Build history of the part. All positions in model axes, mm. A direction names the side the tool comes from. Give positions to 0.01 mm unless a question says otherwise; leave off trailing zeros. Loops run counter-clockwise (first coordinate to the right, second up) from the corner with the lowest first, then second, coordinate; pieces in that order, holes last.
1) Band-saw the part on C-C on x = 26. List the corners of the cut face in (y, z), then the cut area to 3 significant figures.
2) 3-axis set-ups, long thin cutter, end or side, ignore diameter. For faces 1 (the flat face through (5, 27, 5)), 2 (the cylindrical face through (-34.464, -14.013, 1.014)), 3 (the flat face through (-4, -27, 8)): which of +Z, -Z, +X, -X, +Y, -Y reach the whole face in a straight line?
3) Band-saw the part on A-A on y = 0. List the corners of the cut face in (x, z), then the cut area to 3 significant figures.
4) Flat gauge pins, fed straight in: P1, Ø0.7, axis at y = -27.5, z = 4.5, coming from the +X side; P2, Ø3, axis at x = 15.33, y = 32.57, coming from the +Z side; P3, Ø10, axis at x = -13, y = -23.5, coming from the +Z side. Where does each tip first touch, or does it go through?
5) Two-plate mould, pull along X, no slides. Class faces 4 (the flat face through (-2, 22, 9)), 5 (the cylindrical face through (-30.392, 16.864, 1.014)): +X half, -X half, draft (parallel to the pull), parting line (faces both ways), or undercut.
6) Band-saw the part on B-B on x = -7. List the corners of the cut face in (y, z).
7) Wall check: line 1 (Y direction, x = -31, z = 1.5); line 2 (X direction, y = 1, z = 1.5); line 3 (X direction, y = 23.5, z = 4.5). Give the ranges that are in metal, low to high.
```python
from build123d import *

# Parameters (mm, degrees)
SKETCH1_R           = 39
BOSS_EXTRUDE1_DEPTH = 2
SKETCH3_R           = 30.75
BOSS_EXTRUDE2_DEPTH = 5
SKETCH5_R           = 1.7
CUT_EXTRUDE2_DEPTH  = 7
SKETCH6_R           = 3
CUT_EXTRUDE3_DEPTH  = 4.5
SKETCH7_R           = 19
CUT_EXTRUDE4_DEPTH  = 2
SKETCH8_R           = 1.25
CUT_EXTRUDE5_DEPTH  = 2
FILLET1_R           = 1.5
BOSS_EXTRUDE3_DEPTH = 2


with BuildPart() as part:
    # Sketch1 → Boss-Extrude1 (new body)
    with BuildSketch(Plane.XY):
        Circle(SKETCH1_R)
    extrude(amount=BOSS_EXTRUDE1_DEPTH)

    # Sketch3 → Boss-Extrude2 (add)
    with BuildSketch(Plane.XY.offset(2)):
        Circle(SKETCH3_R)
        with BuildLine():
            Line((-5, 26), (-5, 28.311879132))
            ThreePointArc((-5, 28.311879132), (-28.75, 0), (-5, -28.311879132))
            Line((-5, -28.311879132), (-5, -26))
            ThreePointArc((-5, -26), (0, -21), (5, -26))
            Line((5, -26), (5, -28.311879132))
            ThreePointArc((5, -28.311879132), (28.75, 0), (5, 28.311879132))
            Line((5, 28.311879132), (5, 26))
            ThreePointArc((5, 26), (0, 21), (-5, 26))
        make_face(mode=Mode.SUBTRACT)
    extrude(amount=BOSS_EXTRUDE2_DEPTH)

    # Sketch5 → Cut-Extrude2 (cut)
    with BuildSketch(Plane.XY.offset(7)):
        with Locations((0, -26)):
            Circle(SKETCH5_R)
        with Locations((0, 26)):
            Circle(SKETCH5_R)
    extrude(amount=-CUT_EXTRUDE2_DEPTH, mode=Mode.SUBTRACT)

    # Sketch6 → Cut-Extrude3 (cut)
    with BuildSketch(Plane(origin=(0, 0, 0), x_dir=(-1, 0, 0), z_dir=(0, 0, -1))):
        with Locations((0, 26)):
            Circle(SKETCH6_R)
        with Locations((0, -26)):
            Circle(SKETCH6_R)
    extrude(amount=-CUT_EXTRUDE3_DEPTH, mode=Mode.SUBTRACT)

    # Sketch7 → Cut-Extrude4 (cut)
    with BuildSketch(Plane(origin=(0, 0, 0), x_dir=(-1, 0, 0), z_dir=(0, 0, -1))):
        Circle(SKETCH7_R)
    extrude(amount=-CUT_EXTRUDE4_DEPTH, mode=Mode.SUBTRACT)

    # Sketch8 → Cut-Extrude5 (cut)
    with BuildSketch(Plane.XY.offset(2)):
        with Locations((36, 0)):
            Circle(SKETCH8_R)
        with Locations((35.716129247, -4.511996408)):
            Circle(SKETCH8_R)
        with Locations((34.868993801, -8.952835938)):
            Circle(SKETCH8_R)
        with Locations((33.471953492, -13.252483897)):
            Circle(SKETCH8_R)
        with Locations((31.547040482, -17.343132268)):
            Circle(SKETCH8_R)
        with Locations((29.124611797, -21.160269083)):
            Circle(SKETCH8_R)
        with Locations((26.242870587, -24.643695813)):
            Circle(SKETCH8_R)
        with Locations((22.947263631, -27.73847674)):
            Circle(SKETCH8_R)
        with Locations((19.289764619, -30.395805318)):
            Circle(SKETCH8_R)
        with Locations((15.328054496, -32.573773889)):
            Circle(SKETCH8_R)
        with Locations((11.124611797, -34.238034587)):
            Circle(SKETCH8_R)
        with Locations((6.745727325, -35.362341026)):
            Circle(SKETCH8_R)
        with Locations((2.260458703, -35.928962223)):
            Circle(SKETCH8_R)
        with Locations((-2.260458703, -35.928962223)):
            Circle(SKETCH8_R)
        with Locations((-6.745727325, -35.362341026)):
            Circle(SKETCH8_R)
        with Locations((-11.124611797, -34.238034587)):
            Circle(SKETCH8_R)
        with Locations((-15.328054496, -32.573773889)):
            Circle(SKETCH8_R)
        with Locations((-19.289764619, -30.395805318)):
            Circle(SKETCH8_R)
        with Locations((-22.947263631, -27.73847674)):
            Circle(SKETCH8_R)
        with Locations((-26.242870587, -24.643695813)):
            Circle(SKETCH8_R)
        with Locations((-29.124611797, -21.160269083)):
            Circle(SKETCH8_R)
        with Locations((-31.547040482, -17.343132268)):
            Circle(SKETCH8_R)
        with Locations((-33.471953492, -13.252483897)):
            Circle(SKETCH8_R)
        with Locations((-34.868993801, -8.952835938)):
            Circle(SKETCH8_R)
        with Locations((-35.716129247, -4.511996408)):
            Circle(SKETCH8_R)
        with Locations((-36, 0)):
            Circle(SKETCH8_R)
        with Locations((-35.716129247, 4.511996408)):
            Circle(SKETCH8_R)
        with Locations((-34.868993801, 8.952835938)):
            Circle(SKETCH8_R)
        with Locations((-33.471953492, 13.252483897)):
            Circle(SKETCH8_R)
        with Locations((-31.547040482, 17.343132268)):
            Circle(SKETCH8_R)
        with Locations((-29.124611797, 21.160269083)):
            Circle(SKETCH8_R)
        with Locations((-26.242870587, 24.643695813)):
            Circle(SKETCH8_R)
        with Locations((-22.947263631, 27.73847674)):
            Circle(SKETCH8_R)
        with Locations((-19.289764619, 30.395805318)):
            Circle(SKETCH8_R)
        with Locations((-15.328054496, 32.573773889)):
            Circle(SKETCH8_R)
        with Locations((-11.124611797, 34.238034587)):
            Circle(SKETCH8_R)
        with Locations((-6.745727325, 35.362341026)):
            Circle(SKETCH8_R)
        with Locations((-2.260458703, 35.928962223)):
            Circle(SKETCH8_R)
        with Locations((2.260458703, 35.928962223)):
            Circle(SKETCH8_R)
        with Locations((6.745727325, 35.362341026)):
            Circle(SKETCH8_R)
        with Locations((11.124611797, 34.238034587)):
            Circle(SKETCH8_R)
        with Locations((15.328054496, 32.573773889)):
            Circle(SKETCH8_R)
        with Locations((19.289764619, 30.395805318)):
            Circle(SKETCH8_R)
        with Locations((22.947263631, 27.73847674)):
            Circle(SKETCH8_R)
        with Locations((26.242870587, 24.643695813)):
            Circle(SKETCH8_R)
        with Locations((29.124611797, 21.160269083)):
            Circle(SKETCH8_R)
        with Locations((31.547040482, 17.343132268)):
            Circle(SKETCH8_R)
        with Locations((33.471953492, 13.252483897)):
            Circle(SKETCH8_R)
        with Locations((34.868993801, 8.952835938)):
            Circle(SKETCH8_R)
        with Locations((35.716129247, 4.511996408)):
            Circle(SKETCH8_R)
    extrude(amount=-CUT_EXTRUDE5_DEPTH, mode=Mode.SUBTRACT)

    # Fillet1
    # the kernel refuses this fillet: 1.5 mm, written as the material it adds along each edge
    with BuildSketch(Plane(origin=(0, 26, 4.5), x_dir=(-1, 0, 0), z_dir=(0, -1, 0))) as fillet1_piece_1:
        with BuildLine():
            CenterArc((1.5, 1.486606875), FILLET1_R, 277.662255661, 82.337744339)
            Line((1.7, 0), (1.704, -0.029732137))
            ThreePointArc((1.704, -0.029732137), (2.35, -0.03), (3, -0.03))
            Line((3, -0.03), (3.03, 0))
            Line((3.03, 0), (3.03, 1.486606875))
            Line((3.03, 1.486606875), (3, 1.486606875))
        make_face()
    revolve(axis=Axis((0, 26, 4.5), (0, 0, -1)))
    with BuildSketch(Plane(origin=(0, -26, 4.5), x_dir=(-1, 0, 0), z_dir=(0, -1, 0))) as fillet1_piece_2:
        with BuildLine():
            CenterArc((1.5, 1.486606875), FILLET1_R, 277.662255661, 82.337744339)
            Line((1.7, 0), (1.704, -0.029732137))
            ThreePointArc((1.704, -0.029732137), (2.35, -0.03), (3, -0.03))
            Line((3, -0.03), (3.03, 0))
            Line((3.03, 0), (3.03, 1.486606875))
            Line((3.03, 1.486606875), (3, 1.486606875))
        make_face()
    revolve(axis=Axis((0, -26, 4.5), (0, 0, -1)))

    # Sketch9 → Boss-Extrude3 (add)
    with BuildSketch(Plane.XY.offset(7)):
        with BuildLine():
            Line((-4, 28.311879132), (-5, 28.311879132))
            Line((-5, 28.311879132), (-5, 26))
            ThreePointArc((-5, 26), (0, 21), (5, 26))
            Line((5, 26), (5, 28.311879132))
            Line((5, 28.311879132), (4, 28.311879132))
            Line((4, 28.311879132), (4, 26))
            ThreePointArc((4, 26), (0, 22), (-4, 26))
            Line((-4, 26), (-4, 28.311879132))
        make_face()
        with BuildLine():
            Line((-5, -26), (-5, -28.311879132))
            Line((-5, -28.311879132), (-4, -28.311879132))
            Line((-4, -28.311879132), (-4, -26))
            ThreePointArc((-4, -26), (0, -22), (4, -26))
            Line((4, -26), (4, -28.311879132))
            Line((4, -28.311879132), (5, -28.311879132))
            Line((5, -28.311879132), (5, -26))
            ThreePointArc((5, -26), (0, -21), (-5, -26))
        make_face()
    extrude(amount=BOSS_EXTRUDE3_DEPTH)


solid = part.part
```
Findings below:
1. outline: (-29.07, 0) - (-25.87, 0) - (-25.87, 2) - (-29.07, 2) - close; (-23.42, 0) - (23.42, 0) - (23.42, 2) - (16.42, 2) - (16.42, 7) - (12.27, 7) - (12.27, 2) - (-12.27, 2) - (-12.27, 7) - (-16.42, 7) - (-16.42, 2) - (-23.42, 2) - close; (25.87, 0) - (29.07, 0) - (29.07, 2) - (25.87, 2) - close
1. area: 148 mm2
2. face 1: +Z
2. face 2: +Z, -Z
2. face 3: +Z, -Y
3. outline: (-39, 0) - (-37.25, 0) - (-37.25, 2) - (-39, 2) - close; (-34.75, 0) - (-19, 0) - (-19, 2) - (-28.75, 2) - (-28.75, 7) - (-30.75, 7) - (-30.75, 2) - (-34.75, 2) - close; (19, 0) - (34.75, 0) - (34.75, 2) - (30.75, 2) - (30.75, 7) - (28.75, 7) - (28.75, 2) - (19, 2) - close; (37.25, 0) - (39, 0) - (39, 2) - (37.25, 2) - close
3. area: 90.0 mm2
4. P1: stops at x = 14.44
4. P2: stops at z = 2
4. P3: stops at z = 7
5. face 4: draft
5. face 5: undercut
6. outline: (-38.37, 0) - (-36.59, 0) - (-36.59, 2) - (-38.37, 2) - close; (-34.14, 0) - (-17.66, 0) - (-17.66, 2) - (-27.88, 2) - (-27.88, 7) - (-29.94, 7) - (-29.94, 2) - (-34.14, 2) - close; (17.66, 0) - (34.14, 0) - (34.14, 2) - (29.94, 2) - (29.94, 7) - (27.88, 7) - (27.88, 2) - (17.66, 2) - close; (36.59, 0) - (38.37, 0) - (38.37, 2) - (36.59, 2) - close
7. line 1: y = -23.66 to -18.47, -16.22 to 16.22, 18.47 to 23.66
7. line 2: x = -38.99 to -36.75, -35.25 to -18.97, 18.97 to 35.25, 36.75 to 38.99
7. line 3: x = -19.83 to -16.56, -4.33 to 4.33, 16.56 to 19.83
